Could you check a few things on this model? Use its own coordinates, in mm. Face numbers are marked on the shaded views. A direction names the side the tool comes from. Give positions to 0.01 mm unless a question says otherwise; leave off trailing zeros. Order: outer loops, then holes, each group sorted by start corner. A loop starts at its lowest first (then second) coordinate and runs counter-clockwise, first axis right, second up.
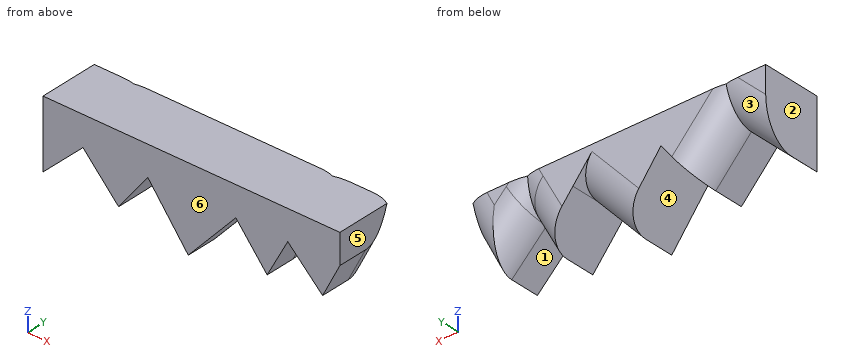
from build123d import *

# Parameters (mm, degrees)
SKETCH1_W           = 127
SKETCH1_H           = 12.7
BOSS_EXTRUDE1_DEPTH = 25.4
BOSS_EXTRUDE2_DEPTH = 25.4
FILLET2_R           = 12.7


with BuildPart() as part:
    # Sketch1 → Boss-Extrude1 (new body)
    with BuildSketch(Plane(origin=(0, 129.522150418, 0), x_dir=(1, 0, 0), z_dir=(0, 1, 0))):
        with Locations((31.151863223, -12.926286206)):
            Rectangle(SKETCH1_W, SKETCH1_H)
    extrude(amount=-BOSS_EXTRUDE1_DEPTH)

    # Sketch2 → Boss-Extrude2 (add)
    with BuildSketch(Plane(origin=(0, 129.522150418, 0), x_dir=(1, 0, 0), z_dir=(0, 1, 0))):
        Polygon((-32.348136777, -6.576286206), (-32.348136777, 9.752049173), (-15.252779509, -6.576286206), (0, 9.752049173), (12.467334528, -6.576286206), (29.798968938, 16.059617503), (50.135874056, -6.576286206), (63.546845791, 9.752049173), (72.350442693, -6.576286206), (87.272954796, 7.906046983), (94.651863223, -6.576286206), (94.651863223, -10.496577103), (-32.348136777, -10.496577103), align=None)
    extrude(amount=-BOSS_EXTRUDE2_DEPTH)

    # Fillet2
    # the kernel refuses this fillet: 12.7 mm, written as the material it takes off along each edge
    with BuildSketch(Plane(origin=(-55.307939563, 129.522150418, -31.681708451), x_dir=(0, -1, 0), z_dir=(0.7231433948257096, 0, 0.6906979300098909))) as fillet2_piece_1_section:
        with BuildLine():
            CenterArc((FILLET2_R, -FILLET2_R), FILLET2_R, 90, 90)
            Line((0, -FILLET2_R), (-FILLET2_R * 0.02, -FILLET2_R))
            Line((-FILLET2_R * 0.02, -FILLET2_R), (-FILLET2_R * 0.02, FILLET2_R * 0.02))
            Line((-FILLET2_R * 0.02, FILLET2_R * 0.02), (FILLET2_R, FILLET2_R * 0.02))
            Line((FILLET2_R, FILLET2_R * 0.02), (FILLET2_R, 0))
        make_face()
    fillet2_piece_1 = extrude(amount=87.140342137, mode=Mode.PRIVATE)
    fillet2_piece_1 = split(fillet2_piece_1, bisect_by=Plane(origin=(-32.348136777, 126.447150631, 1.093343092), z_dir=(1, 0, 0)), keep=Keep.TOP, mode=Mode.PRIVATE)
    fillet2_piece_1 = split(fillet2_piece_1, bisect_by=Plane(origin=(-16.904261861, 126.447150631, 8.344223498), z_dir=(-0.7307649934126457, 0, -0.682629126541357)), keep=Keep.TOP, mode=Mode.PRIVATE)
    add(fillet2_piece_1, mode=Mode.SUBTRACT)
    with BuildSketch(Plane(origin=(-36.926254277, 129.522150418, 29.778074747), x_dir=(0, -1, 0), z_dir=(0.682629126541357, 0, -0.7307649934126457))) as fillet2_piece_2_section:
        with BuildLine():
            CenterArc((FILLET2_R, -FILLET2_R), FILLET2_R, 90, 90)
            Line((0, -FILLET2_R), (-FILLET2_R * 0.02, -FILLET2_R))
            Line((-FILLET2_R * 0.02, -FILLET2_R), (-FILLET2_R * 0.02, FILLET2_R * 0.02))
            Line((-FILLET2_R * 0.02, FILLET2_R * 0.02), (FILLET2_R, FILLET2_R * 0.02))
            Line((FILLET2_R, FILLET2_R * 0.02), (FILLET2_R, 0))
        make_face()
    fillet2_piece_2 = extrude(amount=85.844167449, mode=Mode.PRIVATE)
    fillet2_piece_2 = split(fillet2_piece_2, bisect_by=Plane(origin=(-13.300421888, 126.615006844, 8.441046884), z_dir=(0.6906979300098909, 0, -0.7231433948257096)), keep=Keep.TOP, mode=Mode.PRIVATE)
    fillet2_piece_2 = split(fillet2_piece_2, bisect_by=Plane(origin=(2.843037706, 126.615006844, -6.02855294), z_dir=(-0.7948048188192111, 0, 0.6068651415114903)), keep=Keep.TOP, mode=Mode.PRIVATE)
    add(fillet2_piece_2, mode=Mode.SUBTRACT)
    with BuildSketch(Plane(origin=(72.859080389, 129.522150418, -36.195669189), x_dir=(0, -1, 0), z_dir=(0.45398029626708136, 0, 0.8910117230436719))) as fillet2_piece_3_section:
        with BuildLine():
            CenterArc((FILLET2_R, -FILLET2_R), FILLET2_R, 90, 90)
            Line((0, -FILLET2_R), (-FILLET2_R * 0.02, -FILLET2_R))
            Line((-FILLET2_R * 0.02, -FILLET2_R), (-FILLET2_R * 0.02, FILLET2_R * 0.02))
            Line((-FILLET2_R * 0.02, FILLET2_R * 0.02), (FILLET2_R, FILLET2_R * 0.02))
            Line((FILLET2_R, FILLET2_R * 0.02), (FILLET2_R, 0))
        make_face()
    fillet2_piece_3 = extrude(amount=79.753807682, mode=Mode.PRIVATE)
    fillet2_piece_3 = split(fillet2_piece_3, bisect_by=Plane(origin=(82.345210733, 126.995605854, -3.123659748), z_dir=(0.6964436437658211, 0, 0.7176114903331651)), keep=Keep.TOP, mode=Mode.PRIVATE)
    fillet2_piece_3 = split(fillet2_piece_3, bisect_by=Plane(origin=(94.651863223, 126.995605854, 4.414676038), z_dir=(-1, 0, 0)), keep=Keep.TOP, mode=Mode.PRIVATE)
    add(fillet2_piece_3, mode=Mode.SUBTRACT)
    with BuildSketch(Plane(origin=(49.566277875, 129.522150418, 28.688371895), x_dir=(0, -1, 0), z_dir=(0.7176114903331651, 0, -0.6964436437658211))) as fillet2_piece_4_section:
        with BuildLine():
            CenterArc((FILLET2_R, -FILLET2_R), FILLET2_R, 90, 90)
            Line((0, -FILLET2_R), (-FILLET2_R * 0.02, -FILLET2_R))
            Line((-FILLET2_R * 0.02, -FILLET2_R), (-FILLET2_R * 0.02, FILLET2_R * 0.02))
            Line((-FILLET2_R * 0.02, FILLET2_R * 0.02), (FILLET2_R, FILLET2_R * 0.02))
            Line((FILLET2_R, FILLET2_R * 0.02), (FILLET2_R, 0))
        make_face()
    fillet2_piece_4 = extrude(amount=84.294695045, mode=Mode.PRIVATE)
    fillet2_piece_4 = split(fillet2_piece_4, bisect_by=Plane(origin=(72.424381475, 126.641527383, 6.713423019), z_dir=(0.8802140747510399, 0, -0.4745768458428739)), keep=Keep.TOP, mode=Mode.PRIVATE)
    fillet2_piece_4 = split(fillet2_piece_4, bisect_by=Plane(origin=(90.021052177, 126.641527383, -2.512449501), z_dir=(-0.8910117230436719, 0, 0.45398029626708136)), keep=Keep.TOP, mode=Mode.PRIVATE)
    add(fillet2_piece_4, mode=Mode.SUBTRACT)
    with BuildSketch(Plane(origin=(48.479030935, 129.522150418, -37.698846047), x_dir=(0, -1, 0), z_dir=(0.47457684584287385, 0, 0.8802140747510397))) as fillet2_piece_5_section:
        with BuildLine():
            CenterArc((FILLET2_R, -FILLET2_R), FILLET2_R, 90, 90)
            Line((0, -FILLET2_R), (-FILLET2_R * 0.02, -FILLET2_R))
            Line((-FILLET2_R * 0.02, -FILLET2_R), (-FILLET2_R * 0.02, FILLET2_R * 0.02))
            Line((-FILLET2_R * 0.02, FILLET2_R * 0.02), (FILLET2_R, FILLET2_R * 0.02))
            Line((FILLET2_R, FILLET2_R * 0.02), (FILLET2_R, 0))
        make_face()
    fillet2_piece_5 = extrude(amount=82.050413868, mode=Mode.PRIVATE)
    fillet2_piece_5 = split(fillet2_piece_5, bisect_by=Plane(origin=(59.422424103, 126.616162938, -4.730418982), z_dir=(0.7727631490947523, 0, 0.6346945055703268)), keep=Keep.TOP, mode=Mode.PRIVATE)
    fillet2_piece_5 = split(fillet2_piece_5, bisect_by=Plane(origin=(72.023472886, 126.616162938, 6.893611175), z_dir=(-0.6964436437658211, 0, -0.7176114903331651)), keep=Keep.TOP, mode=Mode.PRIVATE)
    add(fillet2_piece_5, mode=Mode.SUBTRACT)
    with BuildSketch(Plane(origin=(8.579757917, 129.522150418, -39.677567957), x_dir=(0, -1, 0), z_dir=(0.668321606968674, 0, 0.7438724552359828))) as fillet2_piece_6_section:
        with BuildLine():
            CenterArc((FILLET2_R, -FILLET2_R), FILLET2_R, 90, 90)
            Line((0, -FILLET2_R), (-FILLET2_R * 0.02, -FILLET2_R))
            Line((-FILLET2_R * 0.02, -FILLET2_R), (-FILLET2_R * 0.02, FILLET2_R * 0.02))
            Line((-FILLET2_R * 0.02, FILLET2_R * 0.02), (FILLET2_R, FILLET2_R * 0.02))
            Line((FILLET2_R, FILLET2_R * 0.02), (FILLET2_R, 0))
        make_face()
    fillet2_piece_6 = extrude(amount=93.929818377, mode=Mode.PRIVATE)
    fillet2_piece_6 = split(fillet2_piece_6, bisect_by=Plane(origin=(26.326574594, 126.641800239, -11.524512379), z_dir=(0.7939882740207107, 0, 0.6079330725644171)), keep=Keep.TOP, mode=Mode.PRIVATE)
    fillet2_piece_6 = split(fillet2_piece_6, bisect_by=Plane(origin=(49.745548911, 126.641800239, 7.051520961), z_dir=(-0.7727631490947523, 0, -0.6346945055703268)), keep=Keep.TOP, mode=Mode.PRIVATE)
    add(fillet2_piece_6, mode=Mode.SUBTRACT)
    with BuildSketch(Plane(origin=(-55.307939563, 129.522150418, -31.681708451), x_dir=(0, -1, 0), z_dir=(0.7231433948257096, 0, 0.6906979300098909))) as fillet2_piece_7a_section:
        with BuildLine():
            CenterArc((FILLET2_R, -FILLET2_R), FILLET2_R, 90, 90)
            Line((0, -FILLET2_R), (-FILLET2_R * 0.02, -FILLET2_R))
            Line((-FILLET2_R * 0.02, -FILLET2_R), (-FILLET2_R * 0.02, FILLET2_R * 0.02))
            Line((-FILLET2_R * 0.02, FILLET2_R * 0.02), (FILLET2_R, FILLET2_R * 0.02))
            Line((FILLET2_R, FILLET2_R * 0.02), (FILLET2_R, 0))
        make_face()
    fillet2_piece_7a = extrude(amount=87.140342137, mode=Mode.PRIVATE)
    fillet2_piece_7a = split(fillet2_piece_7a, bisect_by=Plane(origin=(-17.333974575, 126.645382706, 8.804237577), z_dir=(0.7307649934126457, 0, 0.682629126541357)), keep=Keep.TOP, mode=Mode.PRIVATE)
    with BuildSketch(Plane(origin=(-36.926254277, 129.522150418, 29.778074747), x_dir=(0, -1, 0), z_dir=(0.682629126541357, 0, -0.7307649934126457))) as fillet2_piece_7b_section:
        with BuildLine():
            CenterArc((FILLET2_R, -FILLET2_R), FILLET2_R, 90, 90)
            Line((0, -FILLET2_R), (-FILLET2_R * 0.02, -FILLET2_R))
            Line((-FILLET2_R * 0.02, -FILLET2_R), (-FILLET2_R * 0.02, FILLET2_R * 0.02))
            Line((-FILLET2_R * 0.02, FILLET2_R * 0.02), (FILLET2_R, FILLET2_R * 0.02))
            Line((FILLET2_R, FILLET2_R * 0.02), (FILLET2_R, 0))
        make_face()
    fillet2_piece_7b = extrude(amount=85.844167449, mode=Mode.PRIVATE)
    fillet2_piece_7b = split(fillet2_piece_7b, bisect_by=Plane(origin=(-13.048064816, 126.645382706, 8.682081385), z_dir=(-0.6906979300098909, 0, 0.7231433948257096)), keep=Keep.TOP, mode=Mode.PRIVATE)
    fillet2_piece_7 = fillet2_piece_7a & fillet2_piece_7b
    add(fillet2_piece_7, mode=Mode.SUBTRACT)
    with BuildSketch(Plane(origin=(49.566277875, 129.522150418, 28.688371895), x_dir=(0, -1, 0), z_dir=(0.7176114903331651, 0, -0.6964436437658211))) as fillet2_piece_8a_section:
        with BuildLine():
            CenterArc((FILLET2_R, -FILLET2_R), FILLET2_R, 90, 90)
            Line((0, -FILLET2_R), (-FILLET2_R * 0.02, -FILLET2_R))
            Line((-FILLET2_R * 0.02, -FILLET2_R), (-FILLET2_R * 0.02, FILLET2_R * 0.02))
            Line((-FILLET2_R * 0.02, FILLET2_R * 0.02), (FILLET2_R, FILLET2_R * 0.02))
            Line((FILLET2_R, FILLET2_R * 0.02), (FILLET2_R, 0))
        make_face()
    fillet2_piece_8a = extrude(amount=84.294695045, mode=Mode.PRIVATE)
    fillet2_piece_8a = split(fillet2_piece_8a, bisect_by=Plane(origin=(86.487490403, 126.688787651, -9.447651295), z_dir=(0.8910117230436719, 0, -0.45398029626708136)), keep=Keep.TOP, mode=Mode.PRIVATE)
    with BuildSketch(Plane(origin=(72.859080389, 129.522150418, -36.195669189), x_dir=(0, -1, 0), z_dir=(0.45398029626708136, 0, 0.8910117230436719))) as fillet2_piece_8b_section:
        with BuildLine():
            CenterArc((FILLET2_R, -FILLET2_R), FILLET2_R, 90, 90)
            Line((0, -FILLET2_R), (-FILLET2_R * 0.02, -FILLET2_R))
            Line((-FILLET2_R * 0.02, -FILLET2_R), (-FILLET2_R * 0.02, FILLET2_R * 0.02))
            Line((-FILLET2_R * 0.02, FILLET2_R * 0.02), (FILLET2_R, FILLET2_R * 0.02))
            Line((FILLET2_R, FILLET2_R * 0.02), (FILLET2_R, 0))
        make_face()
    fillet2_piece_8b = extrude(amount=79.753807682, mode=Mode.PRIVATE)
    fillet2_piece_8b = split(fillet2_piece_8b, bisect_by=Plane(origin=(88.514546729, 126.688787651, -9.111014882), z_dir=(-0.6964436437658211, 0, -0.7176114903331651)), keep=Keep.TOP, mode=Mode.PRIVATE)
    fillet2_piece_8 = fillet2_piece_8a & fillet2_piece_8b
    add(fillet2_piece_8, mode=Mode.SUBTRACT)
    with BuildSketch(Plane(origin=(48.479030935, 129.522150418, -37.698846047), x_dir=(0, -1, 0), z_dir=(0.47457684584287385, 0, 0.8802140747510397))) as fillet2_piece_9a_section:
        with BuildLine():
            CenterArc((FILLET2_R, -FILLET2_R), FILLET2_R, 90, 90)
            Line((0, -FILLET2_R), (-FILLET2_R * 0.02, -FILLET2_R))
            Line((-FILLET2_R * 0.02, -FILLET2_R), (-FILLET2_R * 0.02, FILLET2_R * 0.02))
            Line((-FILLET2_R * 0.02, FILLET2_R * 0.02), (FILLET2_R, FILLET2_R * 0.02))
            Line((FILLET2_R, FILLET2_R * 0.02), (FILLET2_R, 0))
        make_face()
    fillet2_piece_9a = extrude(amount=82.050413868, mode=Mode.PRIVATE)
    fillet2_piece_9a = split(fillet2_piece_9a, bisect_by=Plane(origin=(67.231034688, 126.606396311, 11.544683748), z_dir=(0.6964436437658211, 0, 0.7176114903331651)), keep=Keep.TOP, mode=Mode.PRIVATE)
    with BuildSketch(Plane(origin=(49.566277875, 129.522150418, 28.688371895), x_dir=(0, -1, 0), z_dir=(0.7176114903331651, 0, -0.6964436437658211))) as fillet2_piece_9b_section:
        with BuildLine():
            CenterArc((FILLET2_R, -FILLET2_R), FILLET2_R, 90, 90)
            Line((0, -FILLET2_R), (-FILLET2_R * 0.02, -FILLET2_R))
            Line((-FILLET2_R * 0.02, -FILLET2_R), (-FILLET2_R * 0.02, FILLET2_R * 0.02))
            Line((-FILLET2_R * 0.02, FILLET2_R * 0.02), (FILLET2_R, FILLET2_R * 0.02))
            Line((FILLET2_R, FILLET2_R * 0.02), (FILLET2_R, 0))
        make_face()
    fillet2_piece_9b = extrude(amount=84.294695045, mode=Mode.PRIVATE)
    fillet2_piece_9b = split(fillet2_piece_9b, bisect_by=Plane(origin=(75.736052506, 126.606396311, 12.855693714), z_dir=(-0.8802140747510399, 0, 0.4745768458428739)), keep=Keep.TOP, mode=Mode.PRIVATE)
    fillet2_piece_9 = fillet2_piece_9a & fillet2_piece_9b
    add(fillet2_piece_9, mode=Mode.SUBTRACT)


solid = part.part
Item 1: Imagine slicing it at A-A on y = 115. List the corners of the cut face in (x, z) for me, then the cut area to 3 significant figures.
Findings:
outline: (-32.35, -9.75) - (-15.25, 6.58) - (0, -9.75) - (12.47, 6.58) - (29.8, -16.06) - (50.14, 6.58) - (63.55, -9.75) - (72.35, 6.58) - (87.27, -7.91) - (94.65, 6.58) - (94.65, 19.28) - (-32.35, 19.28) - close
area: 2,750 mm2
Item 2: Imagine slicing it at B-B on x = 51.5. List the corners of the cut face in (y, z) for me, then the cut area to 3 significant figures.
Findings:
outline: (104.12, 4.92) - (129.52, 4.92) - (129.52, 19.28) - (104.12, 19.28) - close
area: 365 mm2
Item 3: For pin 1 (10 mm diameter, centred on y = 114.5, z = 0.5, fed in from +X); pin 2 (8 mm diameter, centred on x = -18.5, z = 7, fed in from +Y); pin 3 (3 mm diameter, centred on y = 111, z = -6.5, fed in from +X), each with a flat end and sliding along its axis, tell me the tip position at first contact or that it passes through.
Findings:
pin 1: stops at x = 94.1
pin 2: stops at y = 127.93
pin 3: stops at x = 88.75
Item 4: Imagine slicing it at C-C on z = -1. Give the number of separate pieces and of enclosed holes in the cut face, then the cut area to 3 significant figures.
Findings:
separate pieces: 5
enclosed holes: 0
area: 1,580 mm2
Item 5: We'd pull the mould along X, two halves only. Please class the marked faces 4, 5 and 6: +X half, -X half, draft (parallel to the pull), parting line (faces both ways), or undercut.
Findings:
face 4: undercut
face 5: +X half
face 6: draft
Item 6: Imagine slicing it at D-D on y = 121.5. List the corners of the cut face in (x, z) for me.
Findings:
outline: (-32.35, -8.52) - (-15.22, 7.85) - (0.55, -9.03) - (12.47, 6.58) - (29.25, -15.34) - (49.56, 7.27) - (62.93, -9.01) - (72.12, 8.04) - (87.03, -6.42) - (94.65, 8.54) - (94.65, 19.28) - (-32.35, 19.28) - close
Item 7: For the marked faces 1, 2 and 3, which set-ups out of +Z, -Z, +X, -X, +Y, -Y let a thin tool reach every point of the face, with its end or its side?
Findings:
face 1: -Z, +Y, -Y
face 2: +Z, -Z, -X, +Y, -Y
face 3: -Z, +Y
Item 8: Please list where these lines run through material, in increasing order: line 1 along X through (y, z) = (108.75, -8.5); line 2 along X through (y, z) = (118.75, -0.5); line 3 along X through (y, z) = (109.25, -3).
Findings:
line 1: x = -32.35 to -31.04, -1.17 to 0.96, 24.01 to 36.59, 62.52 to 64.22
line 2: x = -32.35 to -22.87, -8.44 to 7.06, 17.89 to 43.58, 55.95 to 68.37, 79.85 to 90.88
line 3: x = -32.35 to -25.28, -6.31 to 5.16, 19.8 to 41.53, 58 to 67.19, 82.22 to 89.77
